Autodesk Inventor part; units mm, degrees
ref_plane "Work Plane1" through (5, 0, 0) normal (0, 0.5, 0.866) x (1, 0, 0)
ref_plane "YZ Plane" through (0, 0, 0) normal (1, 0, 0) x (0, 1, 0)
ref_plane "XZ Plane" through (0, 0, 0) normal (0, 1, 0) x (-1, 0, 0)
sketch "Sketch1" plane through (0, 0, 0) normal (0, 0, 1) x (1, 0, 0)
  line L0 (1.0774, 0) -> (10, 0)
  line L1 (10, 0) -> (10, 2)
  line L2 (10, 2) -> (0, 2)
  line L3 (0, 2) -> (0, 3.5)
  line L4 (0, 3.5) -> (-2.8, 3.5)
  line L5 (-2.8, 3.5) -> (-2.8, 1.7321)
  line L6 (-2.8, 1.7321) -> (-1.2, 1.7321)
  line L7 (-1.2, 1.7321) -> (-0.7774, 1)
  line L8 (-5.36, 0) -> (12.56, 0)
  line L9 (0, -0.7) -> (0, 4.2)
  line L10 (-0.7774, 1) -> (0.5, 1)
  line L11 (0.5, 1) -> (1.0774, 0)
  line L12 (-2.8, 1.7321) -> (-2.8, 0) construction
  dimension "d0" = 2.8
  dimension "d1" = 1.6
  dimension "d2" = 60
  dimension "d3" = 4
  dimension "d4" = 3.4641
  dimension "d5" = 7
  dimension "d15" = 3.3
  dimension "d16" = 2
  dimension "d17" = 10
revolve "Body" add sketch "Sketch1" angle 360 about axis through (1.0774, 0, 0) along (1, 0, 0) contours L11 L10 L9 L2 L1 L0 | L10 L7 L6 L5 L4 L3 L9
sketch "Sketch2" plane through (-2.8, 0, 0) normal (-1, 0, 0) x (0, 0, 1)
  circle A0 centre (0, 0) radius 1.7321
  line L0 (0, -4.9) -> (0, 4.9)
  line L1 (-4.9, 0) -> (4.9, 0)
  line L2 (1.7321, 0) -> (0.866, -1.5)
  line L3 (0.866, -1.5) -> (-0.866, -1.5)
  line L4 (-0.866, -1.5) -> (-1.7321, 0)
  line L5 (-1.7321, 0) -> (-0.866, 1.5)
  line L6 (-0.866, 1.5) -> (0.866, 1.5)
  line L7 (0.866, 1.5) -> (1.7321, 0)
extrude "Slot" add sketch "Sketch2" against normal up to next contours L7 A0 | A0 L2 | L6 L0 A0 | A0 L0 L3 | L0 L6 A0 | A0 L3 L0 | L4 A0 | A0 L5
thread "Thread"
chamfer "Chamfer1" distance 0.4294 distance2 0.4294 1 edges at (10, -2, 0) measured on face at (10, 0.556, 0.0273)
ref_plane "Work Plane1" through (5, 0, 0) normal (0, 0.5, 0.866) x (1, 0, 0)
equation "\"d7\" = GEL"
equation "\"d9\" = -0.5 * SPD + 0.5 * GD"
equation "\"d12\" = GUL"
equation "\"d0\" = KOH"
equation "\"d1\" = INTI"
equation "\"d3\" = GD"
equation "\"d4\" = 1.1547 * SW"
equation "\"d5\" = KOD"
equation "\"d15\" = INFT"
equation "\"d16\" = SDT"
equation "\"d17\" = NLG"
equation "\"GD\" = NND"
equation "\"NLG\" = 10"
equation "\"GEL\" = 8"
equation "\"KOD\" = 7"
equation "\"KOH\" = 2.8"
equation "\"GUL\" = 0.61345 * PTC"
equation "\"SW\" = 3"
equation "\"INTI\" = 1.6"
equation "\"SPD\" = NND - 1.2269 * PTC"
equation "\"SDT\" = 2"
equation "\"INFT\" = 3.3"
equation "\"TOA\" = 30deg"
equation "\"GD1\" = THREADDIA - 1.2269 * PTC"
equation "\"THREADDIA\" = 4"
equation "\"BDM\" = NND"
equation "\"RR\" = 0.4"
equation "\"PTC\" = 0.7"
equation "\"NND\" = 4"
equation "\"SLG\" = 2"
equation "\"GAL\" = 0.61345 * PTC"
equation "\"E0\" = 1.155 * SW"
properties part number "CNS 4557 - M4 x 10" material "Steel, Mild"
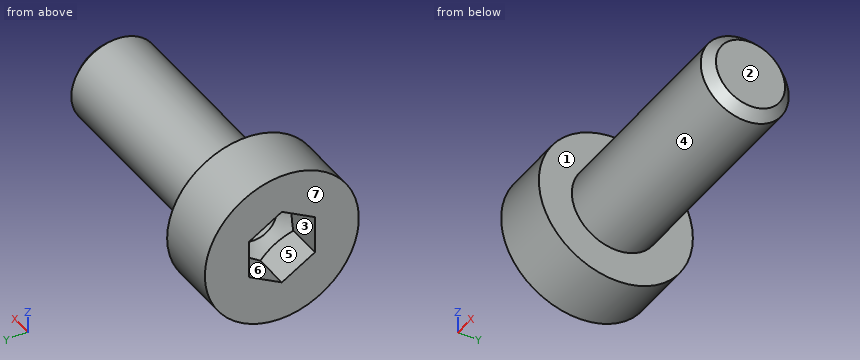
Work out the finished part from the listing and answer in its coordinate system (mm). Face numbers are marked on the shaded views. A direction names the side the tool comes from. Give positions to 0.01 mm unless a question says otherwise; leave off trailing zeros. Loops run counter-clockwise (first coordinate to the right, second up) from the corner with the lowest first, then second, coordinate; pieces in that order, holes last. Notation, with made-up numbers: M 48.25,76.25 L 80.25,76.25 A28 ccw 80.25,111.25 Z; hole C -39.5,89.25 d9. An arc over 180 degrees is marked long. One line per item, written item: value. Start each with the question number.
1. Which of the six approach directions +Z, -Z, +X, -X, +Y, -Y give full straight-line access (tool end or side, diameter ignored) to the marked faces 1, 2 and 3?
2. Find section C-C (z = -3). Give the vertices of the cut face in (x, y), and give its area (3 significant figures).
3. Find the intervals of material crossed by probe 1 along Z at (x, y) = (-0.4, 0); probe 2 along Z at (x, y) = (0.05, 0); probe 3 along X at (y, z) = (3.25, -0.25), in increasing order.
4. Find section B-B (y = 2.25). Give the vertices of the cut face in (x, z), and give its area (3 significant figures).
5. Determine the mould class of the marked faces 4, 5, 6 and 7 for opening direction Z: released by +Z, released by -Z, zero draft, split by the parting line, or undercut.
6. Find section A-A (x = 9.25). Give the vertices of the cut face in (y, z).
7. Each of these flat-tipped pins is pushed along its axis until it touches: P1, Ø0.5, axis at x = -2, z = -0.5, coming from the +Y side; P2, Ø1.5, axis at x = 4.5, y = -1.5, coming from the +Z side; P3, Ø1, axis at x = 5.5, z = 0.5, coming from the -Y side. Where does it stop, or does it pass through?
Reported:
1. face 1: +X
1. face 2: +Z, -Z, +X, +Y, -Y
1. face 3: -X
2. outline: M -2.8,-1.8 L 0,-1.8 L 0,1.8 L -2.8,1.8 Z
2. area: 10.1 mm²
3. probe 1: z = -3.5 to -1, 1 to 3.5
3. probe 2: z = -2 to -1, 1 to 2
3. probe 3: x = -2.8 to 0
4. outline: M -2.8,-2.68 L 0,-2.68 L 0,2.68 L -2.8,2.68 Z
4. area: 15.0 mm²
5. face 4: split by the parting line
5. face 5: undercut
5. face 6: undercut
5. face 7: zero draft
6. outline: C 0,0 d4
7. P1: stops at y = 3.49
7. P2: stops at z = 1.85
7. P3: stops at y = -2
